For this review, take the finished solid that the model builds, in its own axes (mm). Coordinates: 2 decimals unless noted, no trailing zeros. Loops run counter-clockwise (first coordinate to the right, second up) from the corner with the lowest first, then second, coordinate; pieces in that order, holes last.
```python
from build123d import *

# Parameters (mm, degrees)
BOSS_EXTRUDE1_DEPTH = 10
BOSS_EXTRUDE2_DEPTH = 12.7


with BuildPart() as part:
    # Sketch1 → Boss-Extrude1 (new body)
    with BuildSketch(Plane(origin=(0, 0, 0), x_dir=(1, 0, 0), z_dir=(0, 1, 0))):
        Polygon((-248.535594609, 74.707564465), (-221.743927942, -86.042435535), (191.397738725, -86.042435535), (218.189405391, 74.707564465), align=None)
    extrude(amount=BOSS_EXTRUDE1_DEPTH)

    # Sketch2 → Boss-Extrude2 (add)
    with BuildSketch(Plane(origin=(0, 10, 0), x_dir=(1, 0, 0), z_dir=(0, 1, 0))):
        Polygon((-221.743927942, -86.042435535), (191.397738725, -86.042435535), (191.926905391, -82.867435535), (-222.273094609, -82.867435535), align=None)
    extrude(amount=BOSS_EXTRUDE2_DEPTH)


solid = part.part
```
Q1. Consider section A-A (x = -104). State the section outline as (y, z) points.
Q2. The part is to be moulded in two halves that separate along Z. For faces 1 (the face through (-12, 16, 82.867)), 2 (the face through (-18, 10, 3)), 3 (the face through (-18, 11, 86.042)), say which applies: +Z half, -Z half, draft (parallel to the pull), parting line (faces both ways), or undercut.
Q3. Consider section C-C (z = 76.5). State the section outline as (x, y) points.
Q4. Wall thickness on probe 1 along Z at (x, y) = (-56.5, 16.25); probe 2 along Y at (x, z) = (-163, -45); probe 3 along X at (y, z) = (2.25, 49): over which ranges is each line inside the solid? List them lowest first.
Q5. Consider section B-B (y = 17.5). State the section outline as (x, z) points, then the cut area to 3 significant figures.
Q6. For pin 1 Ø2 at (x, z) = (-105.5, -8.5) entering from +Y; pin 2 Ø6.5 at (x, y) = (-78.5, 17.5) entering from -Z; pin 3 Ø1 at (y, z) = (5, -13.5) entering from +X, all flat-tipped, find the tip position at first contact; note any pin that passes through.
Model answer:
1. outline: (0, -74.71) - (10, -74.71) - (10, 82.87) - (22.7, 82.87) - (22.7, 86.04) - (0, 86.04) - close
2. face 1: -Z half
2. face 2: draft
2. face 3: +Z half
3. outline: (-223.33, 0) - (192.99, 0) - (192.99, 10) - (-223.33, 10) - close
4. probe 1: z = 82.87 to 86.04
4. probe 2: y = 0 to 10
4. probe 3: x = -227.92 to 197.57
5. outline: (-222.27, 82.87) - (191.93, 82.87) - (191.4, 86.04) - (-221.74, 86.04) - close
5. area: 1,310 mm2
6. pin 1: stops at y = 10
6. pin 2: stops at z = 82.87
6. pin 3: stops at x = 208.07
